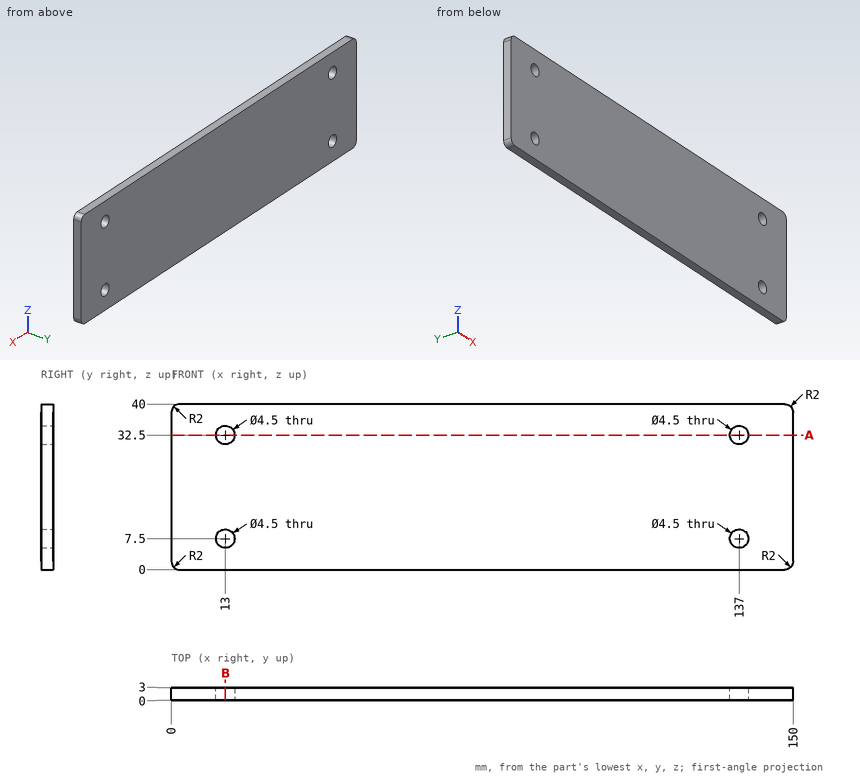
The drawing under review shows one solid part. Ordinate dimensions are in mm from its lowest x, y, z. Give positions to 0.01 mm unless a question says otherwise; leave off trailing zeros. Order: outer loops, then holes, each group sorted by start corner. A loop starts at its lowest first (then second) coordinate and runs counter-clockwise, first axis right, second up. Notation, with made-up numbers: (-35.75, 3) -> (-9.75, 3) arc R14 cw to (-9.75, 15) -> close; hole circle Ø6 at (52, 83). An arc over 180 degrees is marked (long way). Write item = value, one per line. Start each with the question number.
(1) We need section A-A on z = 32.5. Write out the cut boundary in (x, y).
(2) We need section B-B on x = 13. Write out the cut boundary in (y, z), plus the area to 3 significant figures.
(3) For pin 1 (4 mm diameter, centred on x = 137, z = 7.5, fed in from -Y), flat-tipped, find the tip position at first contact; note if it passes through.
(4) To check wall thickness, follow line 1 along X through (y, z) = (1.95, 32.5); line 2 along Z through (x, y) = (137, 1.4); line 3 along X through (y, z) = (0.65, 31). State the ranges of each line that lie inside material, in increasing order.
Numbers:
q1.outline = (0, 0) -> (10.75, 0) -> (10.75, 3) -> (0, 3) -> close; (15.25, 0) -> (134.75, 0) -> (134.75, 3) -> (15.25, 3) -> close; (139.25, 0) -> (150, 0) -> (150, 3) -> (139.25, 3) -> close
q2.outline = (0, 0) -> (3, 0) -> (3, 5.25) -> (0, 5.25) -> close; (0, 9.75) -> (3, 9.75) -> (3, 30.25) -> (0, 30.25) -> close; (0, 34.75) -> (3, 34.75) -> (3, 40) -> (0, 40) -> close
q2.area = 93.0 mm^2
q3.pin_1 = through
q4.line_1 = 0 to 10.75, 15.25 to 134.75, 139.25 to 150
q4.line_2 = 0 to 5.25, 9.75 to 30.25, 34.75 to 40
q4.line_3 = 0 to 11.32, 14.68 to 135.32, 138.68 to 150
